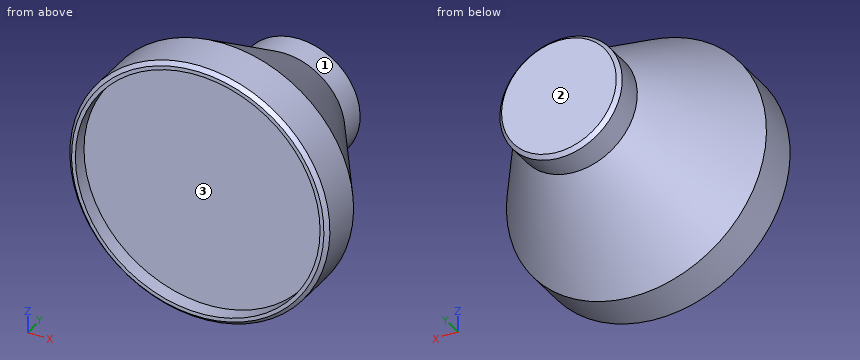
```python
from build123d import *

# Parameters (mm, degrees)
F2_R     = 25.4
F3_DEPTH = 3.175
F4_SIZE  = 0.79375


with BuildPart() as f1:
    # F0 (on Right) → F1 (revolve)
    with BuildSketch(Plane.YZ):
        Polygon((0, 26.9875), (0, 0), (38.1, 0), (38.1, 12.7), (31.75, 12.7), (9.525, 26.9875), align=None)
    revolve(axis=Axis((0, 19.05, 0), (0, -1, 0)))

    # F2 (on face) → F3 (cut)
    with BuildSketch(Plane.XZ):
        Circle(F2_R)
    extrude(amount=-F3_DEPTH, mode=Mode.SUBTRACT)

    # F4
    f4_edges = [f1.edges().sort_by_distance(p)[0] for p in [
        (0, 0, -26.9875),
        (0, 38.1, -12.7),
    ]]
    chamfer(f4_edges, length=F4_SIZE)


solid = f1.part
```
Geometry: final body of the model. Coordinates: model frame, mm. Face numbers are marked on the shaded views. Give positions to 0.01 mm unless a question says otherwise; leave off trailing zeros. Loops run counter-clockwise (first coordinate to the right, second up) from the corner with the lowest first, then second, coordinate; pieces in that order, holes last. Notation, with made-up numbers: (26, 15.5) -> (79, 15.5) arc R25 cw to (79, 34.5) -> close; hole circle Ø2 at (89, -29.5). An arc over 180 degrees is marked (long way). Use one line per item in the form item = value.
Item 1: Pin query (flat end, axial travel): P1, Ø10, axis at x = -16, y = 22, coming from the -Z side; P2, Ø3, axis at x = 0.5, z = 3.5, coming from the -Y side (3 decimals); P3, Ø3, axis at x = -17, y = 19, coming from the -Z side. Return the tip coordinate at first contact, or that it passes through.
A:
P1 = -17.2
P2 = 3.175
P3 = -14.55
Item 2: Section query C-C on y = 36.5. Output: boundary loops of the cut face in (x, z).
A:
outline = circle Ø25.4 at (0, 0)
Item 3: Section query D-D on y = 26.5. Output: boundary loops of the cut face in (x, z) (3 decimals), and give its area (3 significant figures).
A:
outline = circle Ø32.15 at (0, 0)
area = 812 mm^2
Item 4: Line query: probe 1 along Z at (x, y) = (0, 1.85); probe 2 along Z at (x, y) = (-9, 2.5); probe 3 along X at (y, z) = (23.5, 13.5). Output: solid intervals per line, ascending.
A:
probe_1 = -26.99 to -25.4, 25.4 to 26.99
probe_2 = -25.44 to -23.75, 23.75 to 25.44
probe_3 = -11.91 to 11.91
Item 5: Draft query along Z for the marked faces 1, 2 and 3. Return one class per face: pulls with the +Z half, pulls with the -Z half, needs draft (parallel to the pull), parting line crosses it, or undercut.
A:
face_1 = parting line crosses it
face_2 = needs draft
face_3 = undercut
